The figure shows three views and two pictorial views of one solid part (mm, origin at its lowest corner). Answer the questions. A direction names the side the tool comes from. Give positions to 0.01 mm unless a question says otherwise; leave off trailing zeros. Loops run counter-clockwise (first coordinate to the right, second up) from the corner with the lowest first, then second, coordinate; pieces in that order, holes last. Notation, with made-up numbers: M 74.25,-9 L 121.25,-9 A16 cw 121.25,4 Z; hole C -4.5,44.25 d6. An arc over 180 degrees is marked long. Answer in a Markdown table with one row per item. Add a question column.
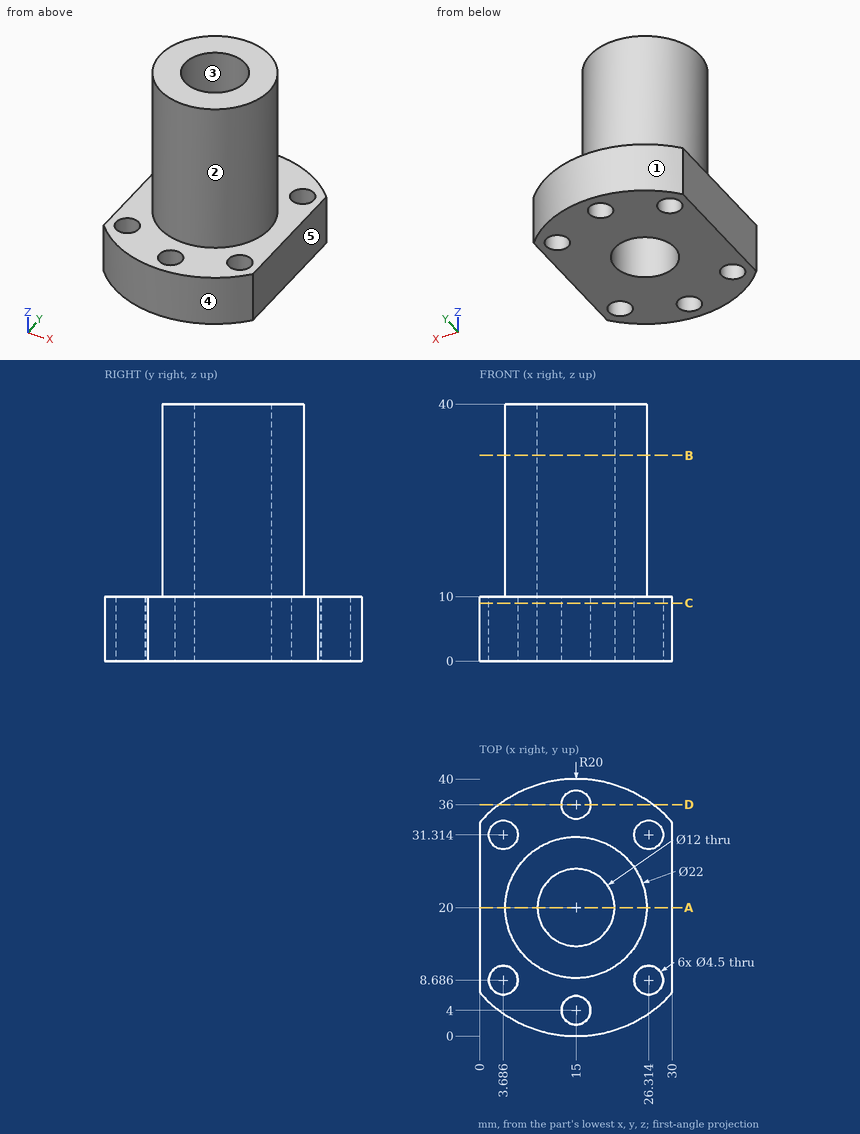
(1) The mould has two halves that part along Y. Classify the marked faces 3, 4 and 5: pulls with the +Y half, pulls with the -Y half, needs draft (parallel to the pull), parting line crosses it, or undercut.
(2) Each of these flat-tipped pins is pushed along its axis until it touches: P1, Ø6, axis at x = 15, y = 36, coming from the +Z side; P2, Ø5, axis at x = 15, y = 4, coming from the -Z side; P3, Ø10, axis at y = 33.5, z = 26.5, coming from the +X side; P4, Ø4, axis at x = 3.69, y = 31.31, coming from the -Z side. Where does it stop, or does it pass through?
(3) Section C-C, the plane z = 9 is taken. Determine the outline of the cut face in (x, y), and give its area (3 significant figures).
(4) Section D-D, the plane y = 36 is taken. Determine the outline of the cut face in (x, z), and give its area (3 significant figures).
(5) Section A-A, the plane y = 20 is taken. Determine the outline of the cut face in (x, z).
(6) Which of the six approach directions +Z, -Z, +X, -X, +Y, -Y give full straight-line access (tool end or side, diameter ignored) to the marked faces 1 and 2?
(7) Section B-B, the plane z = 32 is taken. Determine the outline of the cut face in (x, y), and give its area (3 significant figures).
(8) Consider line 1 along X through (y, z) = (8.5, 6); line 2 along Y through (x, z) = (15, 3.75); line 3 along Y through (x, z) = (16, 7) (1 decimal). Determine where each line is inside the solid, lowest interval first. Write a range as from..to.
Numbers:
| question | item | result |
|---|---|---|
| 1 | face 3 | undercut |
| 1 | face 4 | pulls with the -Y half |
| 1 | face 5 | needs draft |
| 2 | P1 | stops at z = 10 |
| 2 | P2 | stops at z = 0 |
| 2 | P3 | stops at x = 21.98 |
| 2 | P4 | passes through |
| 3 | outline | M 0,6.77 A20 ccw 30,6.77 L 30,33.23 A20 ccw 0,33.23 Z; hole C 3.69,8.69 d4.5; hole C 3.69,31.31 d4.5; hole C 15,20 d12; hole C 15,4 d4.5; hole C 15,36 d4.5; hole C 26.31,8.69 d4.5; hole C 26.31,31.31 d4.5 |
| 3 | area | 867 mm² |
| 4 | outline | M 3,0 L 12.75,0 L 12.75,10 L 3,10 Z; M 17.25,0 L 27,0 L 27,10 L 17.25,10 Z |
| 4 | area | 195 mm² |
| 5 | outline | M 0,0 L 9,0 L 9,40 L 4,40 L 4,10 L 0,10 Z; M 21,0 L 30,0 L 30,10 L 26,10 L 26,40 L 21,40 Z |
| 6 | face 1 | +Z, -Z, +Y |
| 6 | face 2 | +Z |
| 7 | outline | C 15,20 d22; hole C 15,20 d12 |
| 7 | area | 267 mm² |
| 8 | line 1 | x = 0..1.44, 5.93..24.07, 28.56..30 |
| 8 | line 2 | y = 0..1.75, 6.25..14, 26..33.75, 38.25..40 |
| 8 | line 3 | y = 0..2, 6..14.1, 25.9..34, 38..40 |
